from build123d import *

# Parameters (mm, degrees)
SKETCH1_W            = 44
SKETCH1_H            = 30
BOSS_EXTRUDE1_DEPTH  = 54.5
SKETCH5_W            = 5
SKETCH5_H            = 30
BOSS_EXTRUDE3_DEPTH  = 6.8
SKETCH9_R            = 1.35
CUT_EXTRUDE6_DEPTH   = 6
FILLET1_R            = 1.5
FILLET2_R            = 1.25
SKETCH11_W           = 34
SKETCH11_H           = 26
CUT_EXTRUDE7_DEPTH   = 51.25
SKETCH13_R           = 4.05
SKETCH13_R_2         = 1
CUT_EXTRUDE8_DEPTH   = 3.25
CIRPATTERN1_COUNT    = 8
SKETCH15_W           = 20
SKETCH15_H           = 10
CUT_EXTRUDE10_DEPTH  = 5
FILLET6_R            = 1.5
FILLET6_OF_MIRROR4_R = 1.5
SKETCH16_W           = 34
SKETCH16_H           = 44.5
CUT_EXTRUDE11_DEPTH  = 2
FILLET7_R            = 1.25


with BuildPart() as part:
    # Sketch1 → Boss-Extrude1 (new body)
    with BuildSketch(Plane(origin=(0, 0, 0), x_dir=(1, 0, 0), z_dir=(0, 1, 0))):
        with Locations((22, 15)):
            Rectangle(SKETCH1_W, SKETCH1_H)
    extrude(amount=BOSS_EXTRUDE1_DEPTH)

    # Sketch5 → Boss-Extrude3 (add)
    with BuildSketch(Plane(origin=(0, 54.5, 0), x_dir=(1, 0, 0), z_dir=(0, 1, 0))):
        with Locations((2.5, 15)):
            Rectangle(SKETCH5_W, SKETCH5_H)
    boss_extrude3 = extrude(amount=BOSS_EXTRUDE3_DEPTH)

    # Sketch9 → Cut-Extrude6 (cut, through all)
    with BuildSketch(Plane(origin=(5, 0, 0), x_dir=(0, 0, -1), z_dir=(1, 0, 0))):
        with Locations((26, 58.7)):
            Circle(SKETCH9_R)
        with Locations((4, 58.7)):
            Circle(SKETCH9_R)
    cut_extrude6 = extrude(amount=-CUT_EXTRUDE6_DEPTH, mode=Mode.SUBTRACT)

    # Mirror2: Boss-Extrude3, Cut-Extrude6 across plane
    add(boss_extrude3.mirror(Plane.ZY.offset(-22)))
    add(cut_extrude6.mirror(Plane.ZY.offset(-22)), mode=Mode.SUBTRACT)

    # Fillet1
    fillet1_edges = [part.edges().sort_by_distance(p)[0] for p in [
        (2.5, 61.3, 0),
        (2.5, 61.3, -30),
        (41.5, 61.3, -30),
        (41.5, 61.3, 0),
    ]]
    fillet(fillet1_edges, radius=FILLET1_R)

    # Fillet2
    fillet2_edges = [part.edges().sort_by_distance(p)[0] for p in [
        (22, 0, -30),
        (44, 0, -15),
        (22, 0, 0),
        (0, 0, -15),
    ]]
    fillet(fillet2_edges, radius=FILLET2_R)

    # Sketch11 → Cut-Extrude7 (cut)
    with BuildSketch(Plane(origin=(0, 54.5, 0), x_dir=(1, 0, 0), z_dir=(0, 1, 0))):
        with Locations((22, 15)):
            Rectangle(SKETCH11_W, SKETCH11_H)
    extrude(amount=-CUT_EXTRUDE7_DEPTH, mode=Mode.SUBTRACT)

    # Sketch13 → Cut-Extrude8 (cut)
    with BuildSketch(Plane.XZ):
        with Locations((22, -15)):
            Circle(SKETCH13_R)
        with Locations((30, -15)):
            Circle(SKETCH13_R_2)
    cut_extrude8 = extrude(amount=-CUT_EXTRUDE8_DEPTH, mode=Mode.SUBTRACT)

    # CirPattern1: Cut-Extrude8 ×8 about axis
    cirpattern1_axis = Axis((22, 0, -15), (0, 1, 0))
    for i in range(1, CIRPATTERN1_COUNT):
        add(cut_extrude8.rotate(cirpattern1_axis, i * 360 / CIRPATTERN1_COUNT), mode=Mode.SUBTRACT)

    # Sketch15 → Cut-Extrude10 (cut)
    with BuildSketch(Plane(origin=(44, 0, 0), x_dir=(0, 0, -1), z_dir=(1, 0, 0))):
        with Locations((15, 18.25)):
            Rectangle(SKETCH15_W, SKETCH15_H)
        with Locations((15, 40.25)):
            Rectangle(SKETCH15_W, SKETCH15_H)
    cut_extrude10 = extrude(amount=-CUT_EXTRUDE10_DEPTH, mode=Mode.SUBTRACT)

    # Fillet6
    fillet6_edges = [part.edges().sort_by_distance(p)[0] for p in [
        (41.5, 23.25, -5),
        (41.5, 13.25, -5),
        (41.5, 13.25, -25),
        (41.5, 23.25, -25),
        (41.5, 45.25, -5),
        (41.5, 35.25, -5),
        (41.5, 35.25, -25),
        (41.5, 45.25, -25),
    ]]
    fillet(fillet6_edges, radius=FILLET6_R)

    # Mirror4: Cut-Extrude10 across plane
    add(cut_extrude10.mirror(Plane.ZY.offset(-22)), mode=Mode.SUBTRACT)

    # Fillet6 of Mirror4
    fillet6_of_mirror4_edges = [part.edges().sort_by_distance(p)[0] for p in [
        (2.5, 23.25, -5),
        (2.5, 13.25, -5),
        (2.5, 13.25, -25),
        (2.5, 23.25, -25),
        (2.5, 45.25, -5),
        (2.5, 35.25, -5),
        (2.5, 35.25, -25),
        (2.5, 45.25, -25),
    ]]
    fillet(fillet6_of_mirror4_edges, radius=FILLET6_OF_MIRROR4_R)

    # Sketch16 → Cut-Extrude11 (cut)
    with BuildSketch(Plane.XY):
        with Locations((22, 25.5)):
            Rectangle(SKETCH16_W, SKETCH16_H)
    cut_extrude11 = extrude(amount=-CUT_EXTRUDE11_DEPTH, mode=Mode.SUBTRACT)

    # Mirror5: Cut-Extrude11 across plane
    add(cut_extrude11.mirror(Plane(origin=(0, 0, -15), x_dir=(1, 0, 0), z_dir=(0, 0, -1))), mode=Mode.SUBTRACT)

    # Fillet7
    fillet7_edges = [part.edges().sort_by_distance(p)[0] for p in [
        (5, 54.5, -1),
        (5, 47.75, -1),
        (39, 47.75, -1),
        (5, 47.75, -29),
        (39, 47.75, -29),
        (39, 54.5, -1),
        (39, 54.5, -29),
        (5, 54.5, -29),
    ]]
    fillet(fillet7_edges, radius=FILLET7_R)


solid = part.part
Part model, mm, in its own coordinate system. A direction names the side the tool comes from. Coordinates: 2 decimals unless noted, no trailing zeros. Write each loop counter-clockwise with the first axis right and the second up, starting at its lowest first coordinate (ties: lowest second). Pieces come first, ordered by that corner, then holes. Notation, with made-up numbers: M 5.5,-30 L 17.5,-30 A36 cw 17.5,9 Z; hole C 72,82 d10. An arc over 180 degrees is marked long. Return JSON: item names as keys, results as strings.
1. Saw through at C-C, the plane y = 58.7. Write the cut outline in (x, z).
Determined:
{"outline": "M 0,-30 L 5,-30 L 5,-27.35 L 0,-27.35 Z; M 0,-24.65 L 5,-24.65 L 5,-5.35 L 0,-5.35 Z; M 0,-2.65 L 5,-2.65 L 5,0 L 0,0 Z; M 39,-30 L 44,-30 L 44,-27.35 L 39,-27.35 Z; M 39,-24.65 L 44,-24.65 L 44,-5.35 L 39,-5.35 Z; M 39,-2.65 L 44,-2.65 L 44,0 L 39,0 Z"}
2. Flat gauge pins, fed straight in: pin 1 Ø3 at (x, z) = (34.5, -15.5) entering from +Y; pin 2 Ø1 at (x, z) = (21, -29) entering from +Y. Where does each tip first touch, or does it go through?
Determined:
{"pin 1": "y = 3.25", "pin 2": "y = 54.5"}
3. Saw through at A-A, the plane y = 10. Write the cut outline in (x, z), then the cut area to 3 significant figures.
Determined:
{"outline": "M 0,-30 L 5,-30 L 5,0 L 0,0 Z; M 39,-30 L 44,-30 L 44,0 L 39,0 Z", "area": "300 mm²"}
4. Probe L1, parallel to Y at x = 39.5, z = -12.25; L2, parallel to Z at x = 41.2, y = 58.7; L3, parallel to X at y = 25.5, z = -22.5. List the from-to ranges inside material, lowest first.
Determined:
{"L1": "0 to 13.25, 23.25 to 35.25, 45.25 to 61.3", "L2": "-30 to -27.35, -24.65 to -5.35, -2.65 to 0", "L3": "0 to 5, 39 to 44"}
5. 3-axis set-ups, long thin cutter, end or side, ignore diameter. For faces 3 (the face through (16.386, 1.602, -10.342)), 4 (the face through (38.644, 47.374, -1.014)), 5 (the face through (2, 61.3, -15)), 6 (the face through (2.54, 13.7, -5.43)), 7 (the face through (38.644, 54.876, -29.014)): which of +Z, -Z, +X, -X, +Y, -Y reach the whole face in a straight line?
Determined:
{"face 3": "+Y, -Y", "face 4": "+Z, -Z", "face 5": "+Z, -Z, +X, -X, +Y", "face 6": "+X, -X", "face 7": "+Z, -Z, +Y"}
6. Saw through at D-D, the plane x = 22. Write the cut outline in (y, z), then the cut area to 3 significant figures.
Determined:
{"outline": "M 0,-28.75 A1.25 ccw 1.25,-30 L 3.25,-30 L 3.25,-24 L 0,-24 Z; M 0,-22 L 3.25,-22 L 3.25,-19.05 L 0,-19.05 Z; M 0,-10.95 L 3.25,-10.95 L 3.25,-8 L 0,-8 Z; M 0,-6 L 3.25,-6 L 3.25,0 L 1.25,0 A1.25 ccw 0,-1.25 Z; M 47.75,-30 L 54.5,-30 L 54.5,-28 L 47.75,-28 Z; M 47.75,-2 L 54.5,-2 L 54.5,0 L 47.75,0 Z", "area": "84.5 mm²"}
7. Saw through at B-B, the plane x = 30. Write the cut outline in (y, z), then the cut area to 3 significant figures.
Determined:
{"outline": "M 0,-28.75 A1.25 ccw 1.25,-30 L 3.25,-30 L 3.25,-16 L 0,-16 Z; M 0,-14 L 3.25,-14 L 3.25,0 L 1.25,0 A1.25 ccw 0,-1.25 Z; M 47.75,-30 L 54.5,-30 L 54.5,-28 L 47.75,-28 Z; M 47.75,-2 L 54.5,-2 L 54.5,0 L 47.75,0 Z", "area": "117 mm²"}
8. Pull direction X, two halves, no side cores. Call faces 1 (the face through (42, 18, -25)), 2 (the face through (30, 2, -16)): pulls with the +X half, pulls with the -X half, needs draft (parallel to the pull), parting line crosses it, or undercut.
Determined:
{"face 1": "needs draft", "face 2": "undercut"}
